Geometry check sheet. Reference: drawing and pictorial views, mm from the part's lowest x, y, z. A direction names the side the tool comes from. Give positions to 0.01 mm unless a question says otherwise; leave off trailing zeros. Write each loop counter-clockwise with the first axis right and the second up, starting at its lowest first coordinate (ties: lowest second). Pieces come first, ordered by that corner, then holes. Notation, with made-up numbers: (20.25, 6.5) - (58.25, 6.5) arc R37 cw to (58.25, 42.5) - close; hole circle Ø9 at (-39.5, 89). An arc over 180 degrees is marked (long way). Put each result on its own line as item: value.
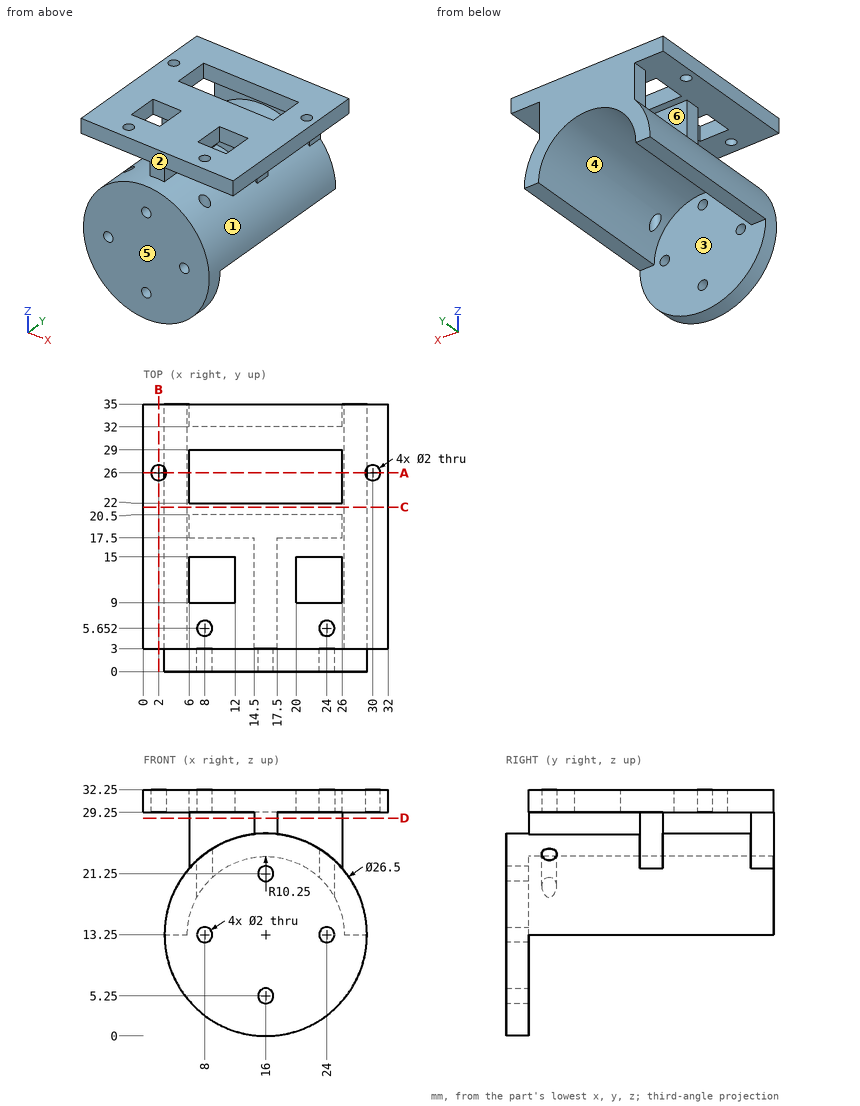
Q1. Section check B-B, the plane x = 2. Record the cut outline in (y, z).
Answers follow:
outline: (3, 29.25) - (25, 29.25) - (25, 32.25) - (3, 32.25) - close; (27, 29.25) - (35, 29.25) - (35, 32.25) - (27, 32.25) - close
Q2. Scan lines: line 1 along Y through (x, z) = (8, 22); line 2 along Y through (x, z) = (2, 31.4); line 3 along Z through (x, y) = (1, 7). Record each from-to range of solid material in increasing order.
Answers follow:
line 1: y = 0 to 4.65, 6.65 to 35
line 2: y = 3 to 25, 27 to 35
line 3: z = 29.25 to 32.25
Q3. Set-up check for the marked faces 4, 5 and 6: record each of +Z, -Z, +X, -X, +Y, -Y from which the full face is reachable in a straight line by a thin tool's end or side.
Answers follow:
face 4: -Z, +Y
face 5: +Z, -Z, +X, -X, -Y
face 6: none
Q4. Section check C-C, the plane y = 21.5. Record the cut outline in (x, z), plus the area to 3 significant figures.
Answers follow:
outline: (0, 29.25) - (32, 29.25) - (32, 32.25) - (0, 32.25) - close; (2.75, 13.25) - (5.75, 13.25) arc R10.25 cw to (26.25, 13.25) - (29.25, 13.25) arc R13.25 ccw to start
area: 207 mm2
Q5. Release check for a two-part mould opening along X. For the marked faces 1, 2 and 3 record: released by +X, released by -X, zero draft, split by the parting line, or undercut.
Answers follow:
face 1: split by the parting line
face 2: zero draft
face 3: undercut
Q6. Section check A-A, the plane y = 26. Record the cut outline in (x, z), plus the area to 3 significant figures.
Answers follow:
outline: (0, 29.25) - (1, 29.25) - (1, 32.25) - (0, 32.25) - close; (2.75, 13.25) - (5.75, 13.25) arc R10.25 cw to (26.25, 13.25) - (29.25, 13.25) arc R13.25 ccw to start; (3, 29.25) - (6, 29.25) - (6, 32.25) - (3, 32.25) - close; (26, 29.25) - (29, 29.25) - (29, 32.25) - (26, 32.25) - close; (31, 29.25) - (32, 29.25) - (32, 32.25) - (31, 32.25) - close
area: 135 mm2
Q7. Section check D-D, the plane z = 28.5. Record the cut outline in (x, y), plus the area to 4 significant figures.
Answers follow:
outline: (6, 17.5) - (14.5, 17.5) - (14.5, 3) - (17.5, 3) - (17.5, 17.5) - (26, 17.5) - (26, 20.5) - (6, 20.5) - close; (6, 32) - (26, 32) - (26, 35) - (6, 35) - close
area: 163.5 mm2
Q8. Go/stop test with flat-tipped pins: pin 1 Ø1.5 at (x, y) = (24.5, 10) entering from -Z; pin 2 Ø4 at (y, z) = (19, 13) entering from -X; pin 3 Ø1 at (x, y) = (7.5, 22) entering from -Z (1 decimal). Record where each tip stops, or that it passes through.
Answers follow:
pin 1: stops at z = 17.67
pin 2: stops at x = 2.75
pin 3: stops at z = 18.2
